Geometry: final body of the model. Coordinates: model frame, mm. A direction names the side the tool comes from. Coordinates: 2 decimals unless noted, no trailing zeros. Order: outer loops, then holes, each group sorted by start corner. A loop starts at its lowest first (then second) coordinate and runs counter-clockwise, first axis right, second up. Notation, with made-up numbers: M 65.5,30.25 L 99.5,30.25 A15 ccw 99.5,56.25 Z; hole C 57.5,34.25 d2. An arc over 180 degrees is marked long. One line per question, with ' | ' between items.
from build123d import *

# Parameters (mm, degrees)
F1_DEPTH = 38.1
F0_R     = 7.9375
F2_DEPTH = 19.05


with BuildPart() as f1:
    # F0 (on Front) → F1 (new body)
    with BuildSketch(Plane.XZ):
        Polygon((-53.922951, 23.130657), (-53.922951, -40.369343), (34.977049, -40.369343), (34.977049, -8.619343), (-9.472951, 23.130657), align=None)
    extrude(amount=F1_DEPTH)

    # F0 (on Front) → F2 (join)
    with BuildSketch(Plane.XZ):
        Polygon((34.977049, -8.619343), (34.977049, -40.369343), (73.077049, -40.369343), (73.077049, -8.619343), (54.027049, -8.619343), align=None)
        with Locations((54.027049, -23.755247)):
            Circle(F0_R, mode=Mode.SUBTRACT)
    extrude(amount=F2_DEPTH)


solid = f1.part
1. Section D-D, the plane y = -35. Output: boundary loops of the cut face in (x, z), and give its area (3 significant figures).
Response values:
outline: M -53.92,-40.37 L 34.98,-40.37 L 34.98,-8.62 L -9.47,23.13 L -53.92,23.13 Z | area: 4,940 mm^2
2. Section A-A, the plane x = 55. Output: boundary loops of the cut face in (y, z).
Response values:
outline: M -19.05,-40.37 L 0,-40.37 L 0,-31.63 L -19.05,-31.63 Z; M -19.05,-15.88 L 0,-15.88 L 0,-8.62 L -19.05,-8.62 Z
3. Pin query (flat end, axial travel): P1, Ø1, axis at x = 42.5, z = -32, coming from the -Y side; P2, Ø15, axis at x = 60.5, y = -10, coming from the +Z side; P3, Ø9.5, axis at y = -29, z = -29, coming from the +X side. Return the tip coordinate at first contact, or that it passes through.
Response values:
P1: stops at y = -19.05 | P2: stops at z = -8.62 | P3: stops at x = 34.98
4. Material intervals for line 1 (X direction, y = -6, z = -30); line 2 (Z direction, x = 55.5, y = -11); line 3 (X direction, y = -32.5, z = -35.5), sorted ascending. Write a range as [from, to].
Response values:
line 1: x = [-53.92, 49.13], [58.93, 73.08] | line 2: z = [-40.37, -31.55], [-15.96, -8.62] | line 3: x = [-53.92, 34.98]
5. Section B-B, the plane y = -10. Output: boundary loops of the cut face in (x, z) (1 decimal), and give its area (3 significant figures).
Response values:
outline: M -53.9,-40.4 L 73.1,-40.4 L 73.1,-8.6 L 35,-8.6 L -9.5,23.1 L -53.9,23.1 Z; hole C 54,-23.8 d15.9 | area: 5,950 mm^2
6. Access query for faces 5 (the face through (54, -9, -8.619)), 6 (the face through (50, -19.05, -31)), 7 (the face through (-10, -38.1, -8)). Directions: +Z, -Z, +X, -X, +Y, -Y. A direction counts if a zero-diameter tool reaches every point of the face in a straight line with its end or side. Return the directions, or none.
Response values:
face 5: +Z, +X, +Y, -Y | face 6: +Z, -Z, +X, -Y | face 7: +Z, -Z, +X, -X, -Y
7. Draft query along Z for faces 1 (the face through (73.077, -9, -25)), 2 (the face through (-31, -19, 23.131)), 3 (the face through (61.359, -9.392, -26.795)), 4 (the face through (-5, -19, -40.369)). Return one class per face: pulls with the +Z half, pulls with the -Z half, needs draft (parallel to the pull), parting line crosses it, or undercut.
Response values:
face 1: needs draft | face 2: pulls with the +Z half | face 3: undercut | face 4: pulls with the -Z half
8. Section C-C, the plane z = -29. Output: boundary loops of the cut face in (x, y), and give its area (3 significant figures).
Response values:
outline: M -53.92,-38.1 L 34.98,-38.1 L 34.98,-19.05 L 48.07,-19.05 L 48.07,0 L -53.92,0 Z; M 59.98,-19.05 L 73.08,-19.05 L 73.08,0 L 59.98,0 Z | area: 3,890 mm^2
